```python
from build123d import *

# Parameters (mm, degrees)
BOSS_EXTRUDE1_DEPTH = 127


with BuildPart() as part:
    # Sketch1 → Boss-Extrude1 (new body)
    with BuildSketch(Plane.XY):
        with BuildLine():
            Line((0, 0), (35.98, 0))
            ThreePointArc((35.98, 0), (37.883814298, 0.788585702), (38.6724, 2.6924))
            Line((38.6724, 2.6924), (38.6724, 36.5252))
            ThreePointArc((38.6724, 36.5252), (33.8972, 41.3004), (29.122, 36.5252))
            ThreePointArc((29.122, 36.5252), (30.4682, 35.179), (31.8144, 36.5252))
            ThreePointArc((31.8144, 36.5252), (33.8972, 38.608), (35.98, 36.5252))
            Line((35.98, 36.5252), (35.98, 2.6924))
            Line((35.98, 2.6924), (0, 2.6924))
            Line((0, 2.6924), (0, 36.5252))
            ThreePointArc((0, 36.5252), (2.0828, 38.608), (4.1656, 36.5252))
            ThreePointArc((4.1656, 36.5252), (5.5118, 35.179), (6.858, 36.5252))
            ThreePointArc((6.858, 36.5252), (2.0828, 41.3004), (-2.6924, 36.5252))
            Line((-2.6924, 36.5252), (-2.6924, 2.6924))
            ThreePointArc((-2.6924, 2.6924), (-1.903814298, 0.788585702), (0, 0))
        make_face()
    extrude(amount=BOSS_EXTRUDE1_DEPTH)


solid = part.part
```
Geometry: final body of the model. Coordinates: model frame, mm. A direction names the side the tool comes from. Round coordinates to 2 decimals unless told otherwise and drop trailing zeros. Order: outer loops, then holes, each group sorted by start corner. A loop starts at its lowest first (then second) coordinate and runs counter-clockwise, first axis right, second up. Notation, with made-up numbers: (85.25, -30.5) -> (141.25, -30.5) arc R28 cw to (141.25, -1.5) -> close; hole circle Ø3 at (-26, 0). An arc over 180 degrees is marked (long way). Use CSV: the item, a comma, the result in double quotes. Start each with the question number.
1) Material intervals for line 1 along X through (y, z) = (20, 120); line 2 along X through (y, z) = (37, 56); line 3 along Y through (x, z) = (7.5, 106.5), sorted ascending. Write a range as from..to.
2) Set-up query: faces 4 (the face through (34, 41.3, 62.6)), 5 (the face through (0, 19, 63)). Return all of +Z, -Z, +X, -X, +Y, -Y with unobstructed straight access to the full face (end or side cutting, diameter ignored); none if empty.
3) Draft query along Y for faces 1 (the face through (2.037, 38.607, 62.611)), 2 (the face through (2.2, 41.3, 62.6)), 3 (the face through (18, 2, 0)). Return one class per face: +Y half, -Y half, draft (parallel to the pull), parting line (faces both ways), or undercut.
4) Section A-A (x = 33). Return the cut outline in (y, z).
5) Section B-B (y = 30.5). Return the cut outline in (x, z).
6) Section D-D (x = 15). Return the cut outline in (y, z), and give its area (3 significant figures).
7) First-contact query: pin 1 Ø10 at (x, y) = (26, 10.5) entering from +Z; pin 2 Ø2 at (x, z) = (7, 112.5) entering from +Y; pin 3 Ø8 at (x, z) = (11.5, 37.5) entering from +Y. Flat tips, straight axial feed; report the tip coordinate or a pass-through.
Returned:
1,line 1,"x = -2.69..0, 35.98..38.67"
1,line 2,"x = -2.67..0.05, 4.11..6.83, 29.15..31.87, 35.93..38.65"
1,line 3,"y = 0..2.69"
2,face 4,"+Z, -Z, +Y"
2,face 5,"+Z, -Z"
3,face 1,"undercut"
3,face 2,"+Y half"
3,face 3,"draft"
4,outline,"(0, 0) -> (2.69, 0) -> (2.69, 127) -> (0, 127) -> close; (38.4, 0) -> (41.22, 0) -> (41.22, 127) -> (38.4, 127) -> close"
5,outline,"(-2.69, 0) -> (0, 0) -> (0, 127) -> (-2.69, 127) -> close; (35.98, 0) -> (38.67, 0) -> (38.67, 127) -> (35.98, 127) -> close"
6,outline,"(0, 0) -> (2.69, 0) -> (2.69, 127) -> (0, 127) -> close"
6,area,"342 mm²"
7,pin 1,"passes through"
7,pin 2,"stops at y = 39.26"
7,pin 3,"stops at y = 2.69"
